Verification items for the finished model (mm, model axes). A direction names the side the tool comes from. Coordinates: 2 decimals unless noted, no trailing zeros. Write each loop counter-clockwise with the first axis right and the second up, starting at its lowest first coordinate (ties: lowest second). Pieces come first, ordered by that corner, then holes.
```python
from build123d import *

# Parameters (mm, degrees)
SKETCH2_W           = 110
SKETCH2_H           = 80
SKETCH2_R           = 1.65
BOSS_EXTRUDE1_DEPTH = 5
SKETCH4_W           = 79
SKETCH4_H           = 27
BOSS_EXTRUDE2_DEPTH = 5
BOSS_EXTRUDE3_DEPTH = 79
SKETCH7_W           = 28
SKETCH7_H           = 22
CUT_EXTRUDE1_DEPTH  = 55.5
CHAMFER1_SIZE       = 10


with BuildPart() as part:
    # Sketch2 → Boss-Extrude1 (new body)
    with BuildSketch(Plane(origin=(0, 0, 0), x_dir=(1, 0, 0), z_dir=(0, 1, 0))):
        Rectangle(SKETCH2_W, SKETCH2_H)
        with Locations(Location((-49, 30, 0), (0, 0, 270))):
            Circle(SKETCH2_R, mode=Mode.SUBTRACT)
        with Locations(Location((-49, 20, 0), (0, 0, 270))):
            Circle(SKETCH2_R, mode=Mode.SUBTRACT)
        with Locations(Location((49, 20, 0), (0, 0, 90))):
            Circle(SKETCH2_R, mode=Mode.SUBTRACT)
        with Locations(Location((49, 30, 0), (0, 0, 90))):
            Circle(SKETCH2_R, mode=Mode.SUBTRACT)
        with Locations(Location((49, -30, 0), (0, 0, 270))):
            Circle(SKETCH2_R, mode=Mode.SUBTRACT)
        with Locations(Location((49, -20, 0), (0, 0, 270))):
            Circle(SKETCH2_R, mode=Mode.SUBTRACT)
        with Locations(Location((-49, -30, 0), (0, 0, 90))):
            Circle(SKETCH2_R, mode=Mode.SUBTRACT)
        with Locations(Location((-49, -20, 0), (0, 0, 90))):
            Circle(SKETCH2_R, mode=Mode.SUBTRACT)
        Polygon((9.5, -11), (9.5, -23), (-9.5, -23), (-9.5, 23), (9.5, 23), (9.5, 11), (37.5, 11), (37.5, -11), align=None, mode=Mode.SUBTRACT)
    extrude(amount=BOSS_EXTRUDE1_DEPTH)

    # Sketch4 → Boss-Extrude2 (add)
    with BuildSketch(Plane(origin=(0, 5, 0), x_dir=(1, 0, 0), z_dir=(0, 1, 0))):
        with Locations((0, 53.5)):
            Rectangle(SKETCH4_W, SKETCH4_H)
        with Locations((0, -53.5)):
            Rectangle(SKETCH4_W, SKETCH4_H)
    extrude(amount=-BOSS_EXTRUDE2_DEPTH)

    # Sketch6 → Boss-Extrude3 (add)
    with BuildSketch(Plane.ZY.offset(39.5)):
        with BuildLine():
            Line((-67, 0), (67, 0))
            ThreePointArc((67, 0), (0, -67), (-67, 0))
        make_face()
    extrude(amount=-BOSS_EXTRUDE3_DEPTH)

    # Sketch7 → Cut-Extrude1 (cut)
    with BuildSketch(Plane(origin=(0, 0, 0), x_dir=(1, 0, 0), z_dir=(0, 1, 0))):
        with Locations((23.5, 0)):
            Rectangle(SKETCH7_W, SKETCH7_H)
        Polygon((-9.5, 23), (-9.5, -23), (9.5, -23), (9.5, -11), (9.5, 11), (9.5, 23), align=None)
    extrude(amount=-CUT_EXTRUDE1_DEPTH, mode=Mode.SUBTRACT)

    # Chamfer1
    chamfer1_edges = [part.edges().sort_by_distance(p)[0] for p in [
        (39.5, -67, 0),
        (-39.5, -67, 0),
        (-39.5, 2.5, -67),
        (39.5, 2.5, -67),
        (39.5, 2.5, 67),
        (-39.5, 2.5, 67),
    ]]
    chamfer(chamfer1_edges, length=CHAMFER1_SIZE)


solid = part.part
```
1. Sectioned sample at B-B, the plane x = 23. Record the boundary of the cut face in (y, z).
2. Gauge pin test, flat ends, axial feed: P1, Ø5.5, axis at x = 44.5, y = 3, coming from the +Z side; P2, Ø5, axis at y = -3, z = 17, coming from the -X side; P3, Ø4, axis at x = -45, y = 2, coming from the -Z side; P4, Ø2.5, axis at x = -49, z = 30, coming from the +Y side. Record the tip position at first contact, or that the pin passes through.
3. Sectioned sample at D-D, the plane z = 30. Give the number of separate pieces and of enclosed holes in the cut face, and give its area (3 significant figures).
4. Sectioned sample at C-C, the plane z = 0. Record the boundary of the cut face in (x, y), and give its area (3 significant figures).
5. Tool access check on faces 4 (the flat face through (47, 0, -1)), 5 (the flat face through (-13, 5, -1)), 6 (the flat face through (9.5, -26, 17)). Record the directions out of +Z, -Z, +X, -X, +Y, -Y that give a thin tool (end or side, any length) a straight path to the whole face; none if there is none.
6. Sectioned sample at A-A, the plane x = 49. Record the boundary of the cut face in (y, z), and give its area (3 significant figures).
7. Draft check along Z on faces 1 (the flat face through (-47, 2, -40)), 2 (the flat face through (-47, 0, -1)), 3 (the flat face through (0, -26, 23)). Enter one of: pulls with the +Z half, pulls with the -Z half, needs draft (parallel to the pull), parting line crosses it, or undercut.
8. Material ranges on L1, parallel to X at y = 2.7, z = -20; L2, parallel to X at y = 3.7, z = -30; L3, parallel to X at y = 2, z = -29, recorded low to high.
Outcome:
1. outline: (-55.5, -11) - (-55.5, 11) - (5, 11) - (5, 67) - (0, 67) arc R67 ccw to (0, -67) - (5, -67) - (5, -11) - close
2. P1: stops at z = 40
2. P2: stops at x = -39.5
2. P3: stops at z = -40
2. P4: passes through
3. separate pieces: 3
3. enclosed holes: 0
3. area: 5,140 mm2
4. outline: (-55, 0) - (-39.5, 0) - (-39.5, -57) - (-29.5, -67) - (29.5, -67) - (39.5, -57) - (39.5, 0) - (55, 0) - (55, 5) - (37.5, 5) - (37.5, -55.5) - (-9.5, -55.5) - (-9.5, 5) - (-55, 5) - close
4. area: 2,900 mm2
5. face 4: +Z, -Z, +X, -Y
5. face 5: +Z, -Z, +X, -X, +Y
5. face 6: +Y
6. outline: (0, -40) - (5, -40) - (5, -31.65) - (0, -31.65) - close; (0, -28.35) - (5, -28.35) - (5, -21.65) - (0, -21.65) - close; (0, -18.35) - (5, -18.35) - (5, 18.35) - (0, 18.35) - close; (0, 21.65) - (5, 21.65) - (5, 28.35) - (0, 28.35) - close; (0, 31.65) - (5, 31.65) - (5, 40) - (0, 40) - close
6. area: 334 mm2
7. face 1: pulls with the -Z half
7. face 2: needs draft
7. face 3: undercut
8. L1: x = -55 to -50.65, -47.35 to -9.5, 9.5 to 47.35, 50.65 to 55
8. L2: x = -55 to -50.65, -47.35 to 47.35, 50.65 to 55
8. L3: x = -55 to -50.31, -47.69 to 47.69, 50.31 to 55
